Autodesk Inventor part; units mm, degrees
ref_plane "YZ Plane" through (0, 0, 0) normal (1, 0, 0) x (0, 1, 0)
ref_plane "XZ Plane" through (0, 0, 0) normal (0, 1, 0) x (-1, 0, 0)
ref_plane "XY Plane" through (0, 0, 0) normal (0, 0, 1) x (1, 0, 0)
sketch "Sketch1" plane through (0, 0, 0) normal (0, 0, 1) x (1, 0, 0)
  circle A0 centre (0, 0) radius 9
  dimension "d0" = 18
extrude "Extrusion1" add sketch "Sketch1" along normal blind 15
sketch "Sketch2" plane through (0, 0, 15) normal (0, 0, 1) x (1, 0, 0)
  circle A0 centre (0, 0) radius 9
  circle A1 centre (0, 0) radius 7
  dimension "d3" = 14
extrude "Extrusion2" cut sketch "Sketch2" against normal blind 13
sketch "Sketch3" plane through (0, 0, 15) normal (0, 0, 1) x (1, 0, 0)
  circle A0 centre (0, 0) radius 7
  circle A1 centre (0, 0) radius 5
  dimension "d6" = 10
extrude "Extrusion3" cut sketch "Sketch3" against normal blind 15 contours A1
properties part number "BUCHA DA PLACA(38)" material "Bronze, Soft Tin"
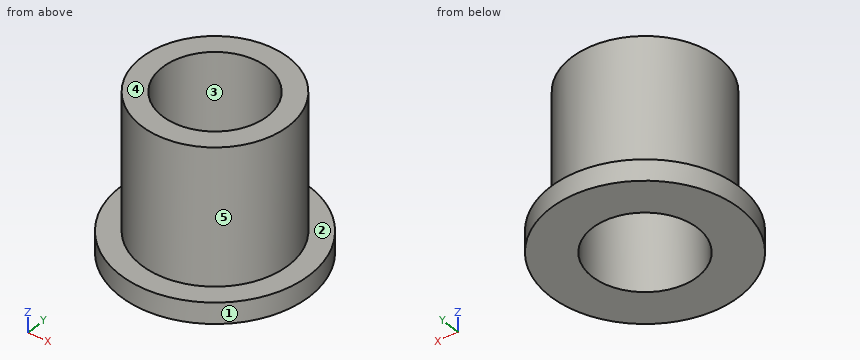
Geometry check sheet. Reference: the model listing, model coordinates, mm. Face numbers are marked on the shaded views. A direction names the side the tool comes from. Coordinates: 2 decimals unless noted, no trailing zeros. Order: outer loops, then holes, each group sorted by start corner. A loop starts at its lowest first (then second) coordinate and runs counter-clockwise, first axis right, second up. Notation, with made-up numbers: (40.25, -24.5) - (50.25, -24.5) arc R16 ccw to (50.25, -19.5) - close; hole circle Ø10 at (71.25, 82.25). An arc over 180 degrees is marked (long way). One line per item, written item: value.
(1) Sectioned sample at A-A (y = 0). Enter the section's corners in (x, z), and give its area (3 significant figures).
Data:
outline: (-9, 0) - (-5, 0) - (-5, 15) - (-7, 15) - (-7, 2) - (-9, 2) - close; (5, 0) - (9, 0) - (9, 2) - (7, 2) - (7, 15) - (5, 15) - close
area: 68.0 mm^2
(2) Release check for a two-part mould opening along Y. For the marked faces 1, 2 and 3 record: +Y half, -Y half, draft (parallel to the pull), parting line (faces both ways), or undercut.
Data:
face 1: parting line
face 2: draft
face 3: undercut
(3) Depth check by flat-ended pin: pin 1 Ø1.5 at (x, z) = (1, 12) entering from +Y; pin 2 Ø6 at (x, z) = (-5.5, 2.5) entering from +Y; pin 3 Ø1.5 at (x, z) = (-6, 7.5) entering from -Y. Enter the tip coordinate at first touch or a pass-through.
Data:
pin 1: stops at y = 7
pin 2: stops at y = 8.63
pin 3: stops at y = -4.63
(4) Sectioned sample at B-B (x = -1.75). Enter the section's corners in (y, z).
Data:
outline: (-8.83, 0) - (-4.68, 0) - (-4.68, 15) - (-6.78, 15) - (-6.78, 2) - (-8.83, 2) - close; (4.68, 0) - (8.83, 0) - (8.83, 2) - (6.78, 2) - (6.78, 15) - (4.68, 15) - close
(5) Sectioned sample at D-D (y = 6.5). Enter the section's corners in (x, z).
Data:
outline: (-6.22, 0) - (6.22, 0) - (6.22, 2) - (2.6, 2) - (2.6, 15) - (-2.6, 15) - (-2.6, 2) - (-6.22, 2) - close
(6) Access from +Z, -Z, +X, -X, +Y, -Y to the whole of each face (thin tool, end or side, straight path). Record for the marked faces 4 and 5.
Data:
face 4: +Z, +X, -X, +Y, -Y
face 5: +Z
(7) Thickness scan on probe 1 along Y at (x, z) = (0, 10); probe 2 along Z at (x, y) = (-4, 6); probe 3 along Y at (x, z) = (3.25, 4.25). Record the ranges inside material, lowest first. Write a range as from..to.
Data:
probe 1: y = -7..-5, 5..7
probe 2: z = 0..2
probe 3: y = -6.2..-3.8, 3.8..6.2
(8) Sectioned sample at C-C (z = 9.5). Enter the section's corners in (x, y), and give its area (3 significant figures).
Data:
outline: circle Ø14 at (0, 0); hole circle Ø10 at (0, 0)
area: 75.4 mm^2
